Geometry: see drawing. Coordinates: mm, zero at the bounding-box minimum. A direction names the side the tool comes from. Give positions to 0.01 mm unless a question says otherwise; leave off trailing zeros. Write each loop counter-clockwise with the first axis right and the second up, starting at its lowest first coordinate (ties: lowest second). Pieces come first, ordered by that corner, then holes. Notation, with made-up numbers: M -16,33 L 6,33 A20 ccw 6,40 Z; hole C -31,51 d7. An arc over 180 degrees is marked long. Use one line per item in the form item = value. Start each with the question number.
Item 1: Section query B-B on z = 13.5. Return loops of the section in (x, y).
Item 2: Pull-direction query (Z, two-part tool) for the marked faces 3, 4 and 5; classes: released by +Z, released by -Z, zero draft, split by the parting line, or undercut.
Item 3: Access query for the marked faces 1 and 2. Directions: +Z, -Z, +X, -X, +Y, -Y. A direction counts if a zero-diameter tool reaches every point of the face in a straight line with its end or side. Return the directions, or none.
Item 4: Section query A-A on y = 16.75. Return loops of the section in (x, z), then the cut area to 3 significant figures.
Item 5: Material intervals for line 1 along X through (y, z) = (23.15, 7.5); line 2 along Y through (x, z) = (14.75, 7); line 3 along X through (y, z) = (5.75, 7.5), sorted ascending. Write a range as from..to.
Item 6: Contact query for flat-ended pins moving along their axis: P1, Ø3, axis at x = 13, z = 6.5, coming from the -Y side; P2, Ø2.5, axis at x = 6, z = 8.5, coming from the -Y side; P3, Ø7, axis at x = 4.5, z = 6.5, coming from the -Y side; P4, Ø5, axis at y = 20, z = 3, coming from the +X side. Output: stop coordinate, or through.
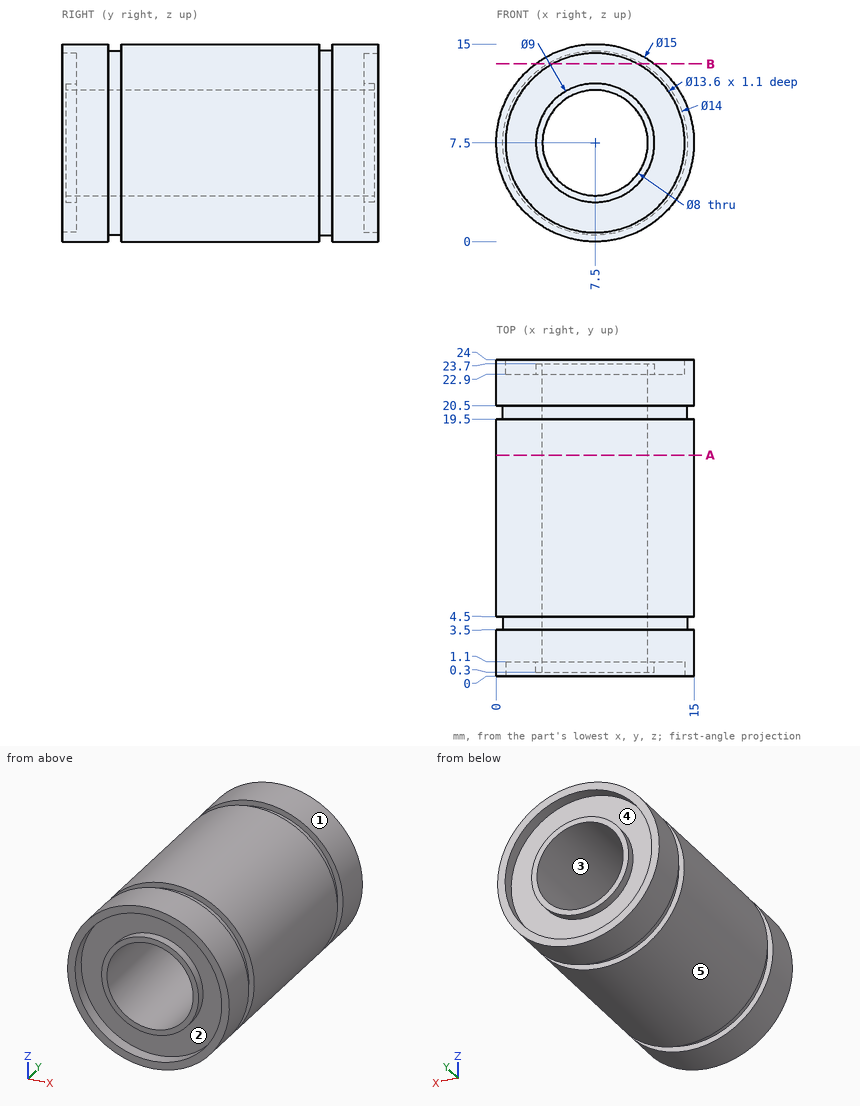
Answer sheet:
q1.outline = M 3,0 L 4.3,0 L 4.3,1.1 L 10.7,1.1 L 10.7,0 L 12,0 L 12,3.5 L 11.11,3.5 L 11.11,4.5 L 12,4.5 L 12,19.5 L 11.11,19.5 L 11.11,20.5 L 12,20.5 L 12,24 L 10.7,24 L 10.7,22.9 L 4.3,22.9 L 4.3,24 L 3,24 L 3,20.5 L 3.89,20.5 L 3.89,19.5 L 3,19.5 L 3,4.5 L 3.89,4.5 L 3.89,3.5 L 3,3.5 Z
q2.face_3 = undercut
q2.face_4 = undercut
q2.face_5 = split by the parting line
q3.face_1 = +Y, -Y
q3.face_2 = -Y
q4.outline = C 7.5,7.5 d15; hole C 7.5,7.5 d8
q4.area = 126 mm2
q5.line_1 = 0..0.7, 3..3.5, 11.5..12, 14.3..15
q5.line_2 = 0..3.5, 4.5..19.5, 20.5..24
q5.line_3 = 0..3.5, 11.5..15
q6.P1 = 0
q6.P2 = through
q6.P3 = 0.3
q6.P4 = 14.71
